Can you work these out from the model? Positions are in its coordinate system, mm. Face numbers are marked on the shaded views. A direction names the side the tool comes from. Round coordinates to 2 decimals unless told otherwise and drop trailing zeros. Loops run counter-clockwise (first coordinate to the right, second up) from the corner with the lowest first, then second, coordinate; pieces in that order, holes last. Notation, with made-up numbers: M 80,12 L 103,12 A14 ccw 103,29 Z; hole C -8.5,85 d10. An arc over 180 degrees is marked long. Return JSON: item names as keys, results as strings.
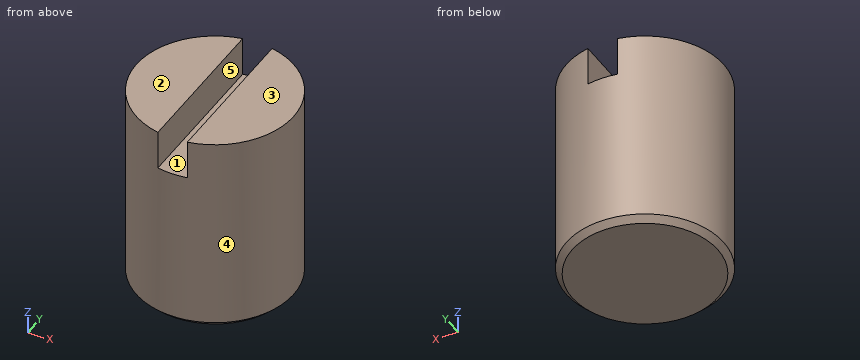
Autodesk Inventor part; units mm, degrees
ref_plane "YZ Plane" through (0, 0, 0) normal (1, 0, 0) x (0, 1, 0)
ref_plane "XZ Plane" through (0, 0, 0) normal (0, 1, 0) x (-1, 0, 0)
ref_plane "XY Plane" through (0, 0, 0) normal (0, 0, 1) x (1, 0, 0)
sketch "Sketch1" plane through (0, 0, 0) normal (0, 0, 1) x (1, 0, 0)
  circle A0 centre (0, 0) radius 4
  dimension "d0" = 8
extrude "Extrusion1" add sketch "Sketch1" along normal blind 10.3
chamfer "Chamfer1" distance 0.3 angle 45 1 edges at (-4, 0, 0)
thread "Thread1"
sketch "Sketch2" plane through (0, 0, 10.3) normal (0, 0, 1) x (1, 0, 0)
  circle A0 centre (0, 0) radius 4
  line L0 (-0.75, -3.9291) -> (-0.75, 3.9291)
  line L1 (0.75, -3.9291) -> (0.75, 3.9291)
  dimension "d7" = 1.5
  dimension "d8" = 0.75
extrude "Extrusion2" cut sketch "Sketch2" against normal blind 2 contours L1 A0 L0
equation "\"d8\" = 0.5 * d7"
properties part number "Terminal Screw" material "Steel, Mild"
Q1. Suppose I cut it at B-B, the plane x = 0. Please give me the cut outline in (y, z).
Results:
{"outline": "M -4,0.3 L -3.7,0 L 3.7,0 L 4,0.3 L 4,8.3 L -4,8.3 Z"}
Q2. Suppose I cut it at A-A, the plane y = 0. Please give me the cut outline in (x, z), plus the area to 3 significant figures.
Results:
{"outline": "M -4,0.3 L -3.7,0 L 3.7,0 L 4,0.3 L 4,10.3 L 0.75,10.3 L 0.75,8.3 L -0.75,8.3 L -0.75,10.3 L -4,10.3 Z", "area": "79.3 mm2"}
Q3. If I drill on line 1 along Y through (x, z) = (-0.75, 5.5); line 2 along X through (y, z) = (-2.25, 8.5); line 3 along X through (y, z) = (-1.25, 9.25), over which ranges is the centre line in solid material (lowest first)?
Results:
{"line 1": "y = -3.93 to 3.93", "line 2": "x = -3.31 to -0.75, 0.75 to 3.31", "line 3": "x = -3.8 to -0.75, 0.75 to 3.8"}
Q4. I'm going to push flat-ended pins straight in: pin 1 Ø1 at (x, y) = (-0.5, -2) entering from -Z; pin 2 Ø0.8 at (x, y) = (0, -1.5) entering from +Z; pin 3 Ø3 at (y, z) = (2.5, 2) entering from +X. Where does each tip first touch, or does it pass through?
Results:
{"pin 1": "stops at z = 0", "pin 2": "stops at z = 8.3", "pin 3": "stops at x = 3.87"}
Q5. On a 3-axis mill with a long thin cutter (end or side, diameter ignored), from which of +Z, -Z, +X, -X, +Y, -Y can I reach the whole of each face in a straight line? I mean the marked faces 1 and 2. Say none if no direction works.
Results:
{"face 1": "+Z, +Y, -Y", "face 2": "+Z, +X, -X, +Y, -Y"}
Q6. Suppose I cut it at C-C, the plane z = 4.25. Please give me the cut outline in (x, y), plus the area to 3 significant figures.
Results:
{"outline": "C 0,0 d8", "area": "50.3 mm2"}
Q7. Thinking about a two-plate mould opening in X: for the marked faces 3, 4 and 5, which applies, pulls with the +X half, pulls with the -X half, needs draft (parallel to the pull), parting line crosses it, or undercut?
Results:
{"face 3": "needs draft", "face 4": "parting line crosses it", "face 5": "undercut"}
